from build123d import *

# Parameters (mm, degrees)
SKETCH1_W           = 20
SKETCH1_H           = 30
BOSS_EXTRUDE1_DEPTH = 65
SKETCH3_R           = 7
CUT_EXTRUDE1_DEPTH  = 60
SKETCH4_R           = 3
CUT_EXTRUDE2_DEPTH  = 21
SKETCH5_W           = 6.5
SKETCH5_H           = 42
CUT_EXTRUDE3_DEPTH  = 31


with BuildPart() as part:
    # Sketch1 → Boss-Extrude1 (new body)
    with BuildSketch(Plane.XY):
        Rectangle(SKETCH1_W, SKETCH1_H)
    extrude(amount=BOSS_EXTRUDE1_DEPTH)

    # Sketch3 → Cut-Extrude1 (cut)
    with BuildSketch(Plane.XY):
        Circle(SKETCH3_R)
    extrude(amount=CUT_EXTRUDE1_DEPTH, mode=Mode.SUBTRACT)

    # Sketch4 → Cut-Extrude2 (cut, through all)
    with BuildSketch(Plane.ZY.offset(10)):
        with Locations((25, 0)):
            Circle(SKETCH4_R)
    extrude(amount=-CUT_EXTRUDE2_DEPTH, mode=Mode.SUBTRACT)

    # Sketch5 → Cut-Extrude3 (cut, through all)
    with BuildSketch(Plane(origin=(0, 15, 0), x_dir=(1, 0, 0), z_dir=(0, 1, 0))):
        with Locations((0, -25)):
            Rectangle(SKETCH5_W, SKETCH5_H)
    extrude(amount=-CUT_EXTRUDE3_DEPTH, mode=Mode.SUBTRACT)


solid = part.part
Read the model definition and answer for the solid it produces. Units are mm, in the model's axes. A direction names the side the tool comes from. Coordinates: 2 decimals unless noted, no trailing zeros. Loops run counter-clockwise (first coordinate to the right, second up) from the corner with the lowest first, then second, coordinate; pieces in that order, holes last. Notation, with made-up numbers: (-1, 58) -> (9, 58) arc R29 cw to (9, 91) -> close; hole circle Ø9 at (23, 37.5). An arc over 180 degrees is marked (long way). Write item = value, one per line. Start each with the question number.
1) The part is cut by section A-A, the plane y = 0. Determine the outline of the cut face in (x, z).
2) The part is cut by section D-D, the plane x = 0. Determine the outline of the cut face in (y, z).
3) Find the intervals of material crossed by L1, parallel to Z at x = -7.1, y = 0; L2, parallel to Y at x = 7.3, z = 25; L3, parallel to X at y = -9, z = 12, in increasing order. Write a range as from..to.
4) For faces 5 (the face through (0, 0, 65)), 6 (the face through (3.763, 5.902, 29.58)), 7 (the face through (0, 11, 4)), determine the directions among +Z, -Z, +X, -X, +Y, -Y from which every point of the face is accessible in a straight line to the end or side of a thin tool.
5) The part is cut by section B-B, the plane z = 5. Determine the outline of the cut face in (x, y).
6) The part is cut by section C-C, the plane z = 25. Determine the outline of the cut face in (x, y).
7) Given P1, Ø1.5, axis at x = 4, y = -3.5, coming from the -Z side, flat-ended and moving along its own axis, determine where the tip first touches the part or whether it passes through.
8) The mould has two halves that part along Z. Classify faces 1 (the face through (-10, 0, 32)), 2 (the face through (-8.19, -1.15, 27.77)), 3 (the face through (-2, 7, 0)), 4 (the face through (3.25, 11, 25)): pulls with the +Z half, pulls with the -Z half, needs draft (parallel to the pull), parting line crosses it, or undercut.
Result:
q1.outline = (-10, 0) -> (-7, 0) -> (-7, 22) -> (-10, 22) -> close; (-10, 28) -> (-7, 28) -> (-7, 60) -> (7, 60) -> (7, 28) -> (10, 28) -> (10, 65) -> (-10, 65) -> close; (7, 0) -> (10, 0) -> (10, 22) -> (7, 22) -> close
q2.outline = (-15, 0) -> (-7, 0) -> (-7, 4) -> (-15, 4) -> close; (-15, 46) -> (-7, 46) -> (-7, 60) -> (7, 60) -> (7, 46) -> (15, 46) -> (15, 65) -> (-15, 65) -> close; (7, 0) -> (15, 0) -> (15, 4) -> (7, 4) -> close
q3.L1 = 0..22, 28..65
q3.L2 = -15..-3, 3..15
q3.L3 = -10..-3.25, 3.25..10
q4.face_5 = +Z, +X, -X, +Y, -Y
q4.face_6 = -Z
q4.face_7 = +Y, -Y
q5.outline = (-10, -15) -> (-3.25, -15) -> (-3.25, -6.2) arc R7 cw to (-3.25, 6.2) -> (-3.25, 15) -> (-10, 15) -> close; (3.25, -15) -> (10, -15) -> (10, 15) -> (3.25, 15) -> (3.25, 6.2) arc R7 cw to (3.25, -6.2) -> close
q6.outline = (-10, -15) -> (-3.25, -15) -> (-3.25, -6.2) arc R7 cw to (-6.32, -3) -> (-10, -3) -> close; (-10, 3) -> (-6.32, 3) arc R7 cw to (-3.25, 6.2) -> (-3.25, 15) -> (-10, 15) -> close; (3.25, -15) -> (10, -15) -> (10, -3) -> (6.32, -3) arc R7 cw to (3.25, -6.2) -> close; (3.25, 6.2) arc R7 cw to (6.32, 3) -> (10, 3) -> (10, 15) -> (3.25, 15) -> close
q7.P1 = 60
q8.face_1 = needs draft
q8.face_2 = undercut
q8.face_3 = pulls with the -Z half
q8.face_4 = undercut
